```python
from build123d import *

# Parameters (mm, degrees)
F1_DEPTH = 7.5
F2_W     = 5
F2_H     = 5
F3_DEPTH = 36.0419135764
F5_DEPTH = 39.3407459622
F6_R     = 3
F7_DEPTH = 56.9630184207


with BuildPart() as f1:
    # F0 (on Front) → F1 (new body, symmetric)
    with BuildSketch(Plane.XZ):
        with BuildLine():
            Line((-5.3623111018, -4.4995132678), (-15.0041252471, 6.991153379))
            Line((-15.0041252471, 6.991153379), (-17.3022585765, 5.0627905499))
            Line((-17.3022585765, 5.0627905499), (-4.6630765815, -10))
            Line((-4.6630765815, -10), (25, -10))
            ThreePointArc((25, -10), (27.588190451, -10.3407417371), (30, -11.3397459622))
            Line((30, -11.3397459622), (90.6217782649, -46.3397459622))
            Line((90.6217782649, -46.3397459622), (92.1217782649, -43.7416697508))
            Line((92.1217782649, -43.7416697508), (28.4833395016, -7))
            Line((28.4833395016, -7), (0, -7))
            ThreePointArc((0, -7), (-2.9583278322, -6.3441545093), (-5.3623111018, -4.4995132678))
        make_face()
    extrude(amount=F1_DEPTH, both=True)

    # F2 (on face) → F3 (cut, through all)
    with BuildSketch(Plane(origin=(-5.3623111018, 0, -4.4995132678), x_dir=(0, 1, 0), z_dir=(0.7660444431, 0, 0.6427876097))):
        with BuildLine():
            ThreePointArc((-7.5, 7.5), (-5.3033008589, 12.8033008589), (0, 15))
            Line((0, 15), (-7.5, 15))
            Line((-7.5, 15), (-7.5, 7.5))
        make_face()
        with Locations((0, 7.5)):
            Rectangle(F2_W, F2_H)
        with BuildLine():
            ThreePointArc((0, 15), (5.3033008589, 12.8033008589), (7.5, 7.5))
            Line((7.5, 7.5), (7.5, 15))
            Line((7.5, 15), (0, 15))
        make_face()
    extrude(amount=-F3_DEPTH, mode=Mode.SUBTRACT)

    # F4 (on face) → F5 (cut, through all)
    with BuildSketch(Plane.XY.offset(-7)):
        with BuildLine():
            ThreePointArc((7.2416697508, 4), (3.2416697508, 0), (7.2416697508, -4))
            Line((7.2416697508, -4), (21.2416697508, -4))
            ThreePointArc((21.2416697508, -4), (25.2416697508, 0), (21.2416697508, 4))
            Line((21.2416697508, 4), (7.2416697508, 4))
        make_face()
    extrude(amount=-F5_DEPTH, mode=Mode.SUBTRACT)

    # F6 (on face) → F7 (cut, through all)
    with BuildSketch(Plane(origin=(4.0897459622, 0, 7.0836477965), x_dir=(0.8660254038, 0, -0.5), z_dir=(0.5, 0, 0.8660254038))):
        with Locations((39.1506350946, 0)):
            Circle(F6_R)
        with Locations((94.1506350946, 0)):
            Circle(F6_R)
        with BuildLine():
            ThreePointArc((94.1506350946, 7.5), (99.4539359535, 5.3033008589), (101.6506350946, 0))
            Line((101.6506350946, 0), (101.6506350946, 7.5))
            Line((101.6506350946, 7.5), (94.1506350946, 7.5))
        make_face()
        with BuildLine():
            ThreePointArc((101.6506350946, 0), (99.4539359535, -5.3033008589), (94.1506350946, -7.5))
            Line((94.1506350946, -7.5), (101.6506350946, -7.5))
            Line((101.6506350946, -7.5), (101.6506350946, 0))
        make_face()
    extrude(amount=-F7_DEPTH, mode=Mode.SUBTRACT)


solid = f1.part
```
Source: CAD feature listing. Evaluate the final solid. Frame: model axes, mm. A direction names the side the tool comes from. Round coordinates to 2 decimals unless told otherwise and drop trailing zeros. Order: outer loops, then holes, each group sorted by start corner. A loop starts at its lowest first (then second) coordinate and runs counter-clockwise, first axis right, second up. Notation, with made-up numbers: (3.5, 69.25) -> (16.5, 69.25) arc R27 ccw to (16.5, 102.25) -> close; hole circle Ø1 at (-25.75, -5.75). An arc over 180 degrees is marked (long way). Use CSV: the item, a comma, the result in double quotes.
(1) Access query for faces 1 (the face through (-9.71, -0.03, -1.62)), 2 (the face through (14, -5, -7)), 3 (the face through (-11, -2.5, 0)). Directions: +Z, -Z, +X, -X, +Y, -Y. A direction counts if a zero-diameter tool reaches every point of the face in a straight line with its end or side. Return the directions, or none.
Report:
face 1,"+Z, -X"
face 2,"+Z, +X, +Y, -Y"
face 3,"none"
(2) Ray query, L1, parallel to Z at x = 4, y = 4.25; L2, parallel to Z at x = -5, y = 4; L3, parallel to X at y = 3, z = -19.5. Return the intervals inside material, ascending.
Report:
L1,"-10 to -7"
L2,"-9.6 to -4.9"
L3,"44.13 to 50.13"
(3) Pull-direction query (Y, two-part tool) for faces 4 (the face through (3, 2, -10)), 5 (the face through (36, 7.5, -14)), 6 (the face through (82.83, -1.83, -40.08)); classes: +Y half, -Y half, draft (parallel to the pull), parting line (faces both ways), or undercut.
Report:
face 4,"draft"
face 5,"+Y half"
face 6,"undercut"
(4) Section D-D on x = 77.5. Return the cut outline in (y, z).
Report:
outline,"(-7.5, -38.76) -> (7.5, -38.76) -> (7.5, -35.3) -> (-7.5, -35.3) -> close"
(5) Section A-A on y = 0. Return the cut outline in (x, z).
Report:
outline,"(-17.3, 5.06) -> (-14.09, 1.23) -> (-11.79, 3.16) -> (-15, 6.99) -> close; (-10.87, -2.6) -> (-4.66, -10) -> (3.24, -10) -> (3.24, -7) -> (0, -7) arc R7 cw to (-5.36, -4.5) -> (-8.58, -0.67) -> close; (25.24, -10) arc R10 cw to (30, -11.34) -> (33.9, -13.59) -> (35.4, -10.99) -> (28.48, -7) -> (25.24, -7) -> close; (39.09, -16.59) -> (81.53, -41.09) -> (83.03, -38.49) -> (40.59, -13.99) -> close; (86.72, -44.09) -> (90.62, -46.34) -> (92.12, -43.74) -> (88.22, -41.49) -> close"
(6) Section B-B on y = -5. Return the cut outline in (x, z), and give its area (3 significant figures).
Report:
outline,"(-16.07, 3.6) -> (-4.66, -10) -> (25, -10) arc R10 cw to (30, -11.34) -> (88.97, -45.38) -> (90.47, -42.79) -> (28.48, -7) -> (0, -7) arc R7 cw to (-5.36, -4.5) -> (-13.78, 5.53) -> close"
area,"363 mm^2"
(7) Section C-C on z = -31. Return the cut outline in (x, y), and give its area (3 significant figures).
Report:
outline,"(64.05, -7.5) -> (70.05, -7.5) -> (70.05, 7.5) -> (64.05, 7.5) -> close"
area,"90.0 mm^2"
(8) First-contact query: pin 1 Ø1 at (x, y) = (22, -3.5) entering from -Z; pin 2 Ø1.5 at (y, z) = (-5.5, -19) entering from -X; pin 3 Ø3 at (x, y) = (15, -4.5) entering from +Z. Flat tips, straight axial feed; report the tip coordinate or a pass-through.
Report:
pin 1,"z = -10"
pin 2,"x = 41.97"
pin 3,"z = -7"
